The listing builds one solid part. Answer for the finished solid, in the listing's coordinates (mm). Face numbers are marked on the shaded views. Coordinates: 2 decimals unless noted, no trailing zeros. Loops run counter-clockwise (first coordinate to the right, second up) from the corner with the lowest first, then second, coordinate; pieces in that order, holes last. Notation, with made-up numbers: M 19,43.5 L 71,43.5 A9 ccw 71,53.5 Z; hole C 73,-22 d9. An arc over 180 degrees is marked long. Return JSON: item names as keys, results as strings. Group by question number.
1. Section B-B (z = 1.8) is taken. Count the separate pieces of the cut face and the enclosed holes in it, then the cut area to 3 significant figures.
2. Section A-A (y = 0) is taken. Write down the section's boundary in (x, z), then the cut area to 3 significant figures.
3. Straight lines are drawn through the part: L1, parallel to X at y = 48, z = 1.9; L2, parallel to X at y = 22.5, z = 1; L3, parallel to X at y = 73.5, z = 2.15. For each, find the intervals that lie inside material, in ascending order. Write a range as from..to.
4. Given P1, Ø1.5, axis at y = 73, z = 2, coming from the -X side; P2, Ø1.5, axis at y = 11, z = 2.5, coming from the +X side; P3, Ø1, axis at y = 10, z = 3.5, coming from the +X side, each flat-ended and moving along its own axis, determine where each tip first touches the part or whether it passes through.
5. The mould has two halves that part along Y. Classify the marked faces 1, 2 and 3: pulls with the +Y half, pulls with the -Y half, needs draft (parallel to the pull), parting line crosses it, or undercut.
6. Section C-C (x = -14.5) is taken. Write down the section's boundary in (y, z), then the cut area to 3 significant figures.
7. Section D-D (y = 77) is taken. Write down the section's boundary in (x, z), then the cut area to 3 significant figures.
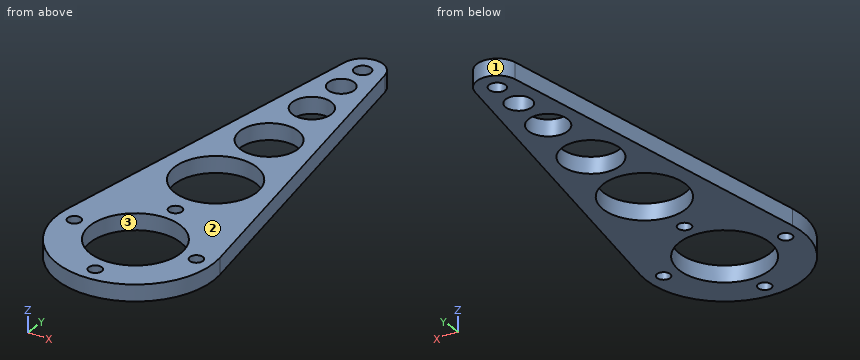
```python
from build123d import *

# Parameters (mm, degrees)
ESQUISSE1_R        = 1.6
ESQUISSE1_R_2      = 11
ESQUISSE1_R_3      = 2
ESQUISSE1_R_4      = 3.163636364
ESQUISSE1_R_5      = 10
ESQUISSE1_R_6      = 7.090909091
ESQUISSE1_R_7      = 4.763636364
BOSS_EXTRU_1_DEPTH = 4


with BuildPart() as part:
    # Esquisse1 → Boss.-Extru.1 (new body)
    with BuildSketch(Plane.XY):
        with BuildLine():
            Line((-18.740511786, 3.129411765), (-4.931713628, 85.823529412))
            ThreePointArc((-4.931713628, 85.823529412), (0, 90), (4.931713628, 85.823529412))
            Line((4.931713628, 85.823529412), (18.740511786, 3.129411765))
            ThreePointArc((18.740511786, 3.129411765), (0, -19), (-18.740511786, 3.129411765))
        make_face()
        with Locations((0, 15)):
            Circle(ESQUISSE1_R, mode=Mode.SUBTRACT)
        with Locations((15, 0)):
            Circle(ESQUISSE1_R, mode=Mode.SUBTRACT)
        with Locations((0, -15)):
            Circle(ESQUISSE1_R, mode=Mode.SUBTRACT)
        with Locations((-15, 0)):
            Circle(ESQUISSE1_R, mode=Mode.SUBTRACT)
        Circle(ESQUISSE1_R_2, mode=Mode.SUBTRACT)
        with Locations((0, 85)):
            Circle(ESQUISSE1_R_3, mode=Mode.SUBTRACT)
        with Locations((0, 77)):
            Circle(ESQUISSE1_R_4, mode=Mode.SUBTRACT)
        with Locations((0, 30)):
            Circle(ESQUISSE1_R_5, mode=Mode.SUBTRACT)
        with Locations((0, 50)):
            Circle(ESQUISSE1_R_6, mode=Mode.SUBTRACT)
        with Locations((0, 66)):
            Circle(ESQUISSE1_R_7, mode=Mode.SUBTRACT)
    extrude(amount=BOSS_EXTRU_1_DEPTH)


solid = part.part
```
Worked out:
{
 "1": {"separate pieces": "1", "enclosed holes": "10", "area": "1,670 mm^2"},
 "2": {"outline": "M -19,0 L -16.6,0 L -16.6,4 L -19,4 Z; M -13.4,0 L -11,0 L -11,4 L -13.4,4 Z; M 11,0 L 13.4,0 L 13.4,4 L 11,4 Z; M 16.6,0 L 19,0 L 19,4 L 16.6,4 Z", "area": "38.4 mm^2"},
 "3": {"L1": "-11.25..-6.8, 6.8..11.25", "L2": "-15.51..-6.61, 6.61..15.51", "L3": "-6.99..6.99"},
 "4": {"P1": "x = -7.2", "P2": "x = 17.55", "P3": "x = 17.68"},
 "5": {"face 1": "pulls with the +Y half", "face 2": "needs draft", "face 3": "undercut"},
 "6": {"outline": "M -12.28,0 L -1.52,0 L -1.52,4 L -12.28,4 Z; M 1.52,0 L 28.52,0 L 28.52,4 L 1.52,4 Z", "area": "151 mm^2"},
 "7": {"outline": "M -6.41,0 L -3.16,0 L -3.16,4 L -6.41,4 Z; M 3.16,0 L 6.41,0 L 6.41,4 L 3.16,4 Z", "area": "25.9 mm^2"}
}
